Design review of the part shown in the three views and the two pictorial views. Dimensions are in mm from the part's minimum x, y and z. A direction names the side the tool comes from. Give positions to 0.01 mm unless a question says otherwise; leave off trailing zeros. Order: outer loops, then holes, each group sorted by start corner. A loop starts at its lowest first (then second) coordinate and runs counter-clockwise, first axis right, second up. Notation, with made-up numbers: (79.25, 13.5) -> (124.25, 13.5) arc R19 ccw to (124.25, 21.5) -> close; hole circle Ø11 at (70, 71). An arc over 180 degrees is marked (long way). Answer in a Markdown table with one row per item. Add a question column.
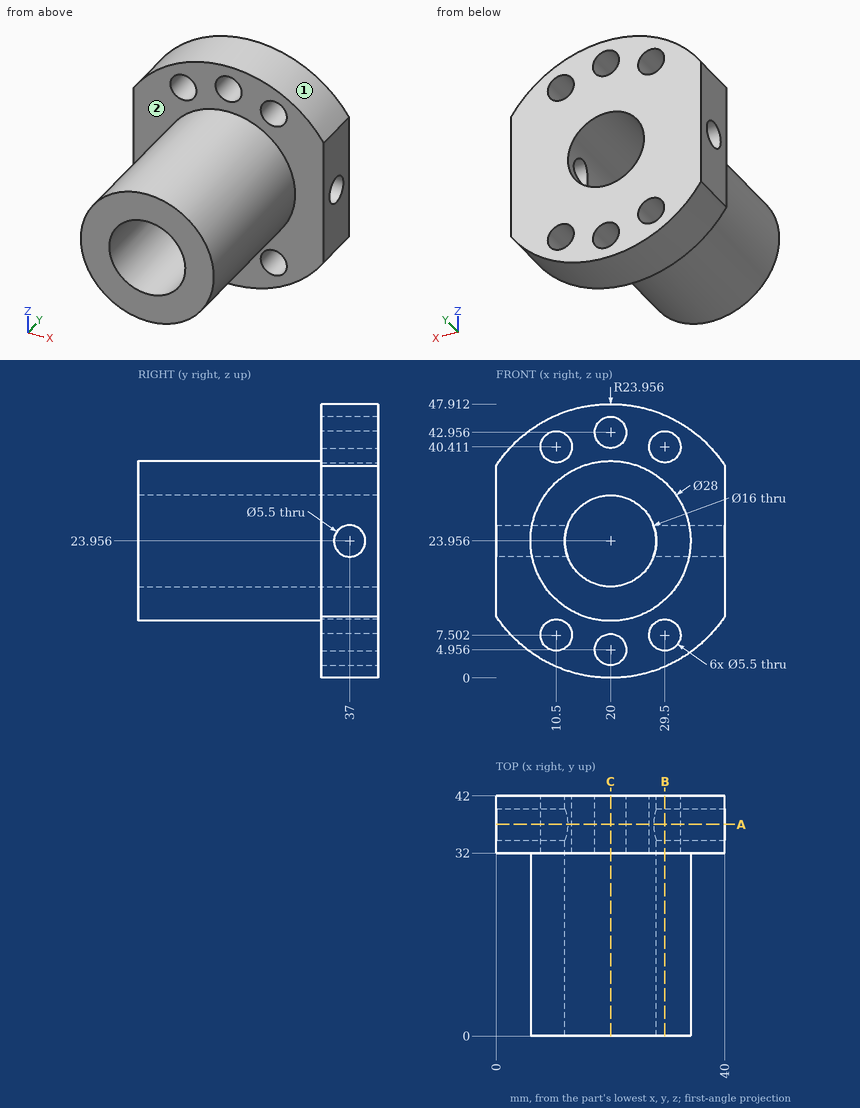
1) Add section A-A, the plane y = 37. Write out the cut boundary in (x, z), and give its area (3 significant figures).
2) For L1, parallel to Z at x = 10, y = 35 (1 decimal); L2, parallel to X at y = 24.5, z = 24.5; L3, parallel to Z at x = 22, y = 12, list the stretches that pass through material, from the lowest coordinate up.
3) Clearance check with flat-ended pins moving along their axes: P1, Ø8, axis at x = 16.5, z = 27, coming from the +Y side; P2, Ø10, axis at y = 10, z = 9.5, coming from the +X side (1 decimal); P3, Ø14.5, axis at x = 20, z = 23.96, coming from the +Y side; P4, Ø6, axis at x = 30, y = 9, coming from the -Z side. State where each tip first meets the part, or that it passes through.
4) Add section C-C, the plane x = 20. Write out the cut boundary in (y, z), and give its area (3 significant figures).
5) Machinability: for the marked faces 1 and 2, which of the approach directions +Z, -Z, +X, -X, +Y, -Y give a long, thin tool a straight path to every point of the face, cutting with its end or side? Answer none if there is none.
6) Add section B-B, the plane x = 29.5. Give the number of separate pieces and of enclosed holes in the cut face, and give its area (3 significant figures).
Verdict:
| question | item | result |
|---|---|---|
| 1 | outline | (0, 10.77) arc R23.96 ccw to (40, 10.77) -> (40, 21.21) -> (27.51, 21.21) arc R8 cw to (12.49, 21.21) -> (0, 21.21) -> close; (0, 26.71) -> (12.49, 26.71) arc R8 cw to (27.51, 26.71) -> (40, 26.71) -> (40, 37.14) arc R23.96 ccw to (0, 37.14) -> close; hole circle Ø5.5 at (10.5, 7.5); hole circle Ø5.5 at (10.5, 40.41); hole circle Ø5.5 at (20, 4.96); hole circle Ø5.5 at (20, 42.96); hole circle Ø5.5 at (29.5, 7.5); hole circle Ø5.5 at (29.5, 40.41) |
| 1 | area | 1,180 mm2 |
| 2 | L1 | z = 2.2 to 4.8, 10.2 to 22.1, 25.8 to 37.7, 43.1 to 45.7 |
| 2 | L2 | x = 6.01 to 12.02, 27.98 to 33.99 |
| 2 | L3 | z = 10.1 to 16.21, 31.7 to 37.81 |
| 3 | P1 | stops at y = 42 |
| 3 | P2 | stops at x = 30.3 |
| 3 | P3 | passes through |
| 3 | P4 | stops at z = 11.83 |
| 4 | outline | (0, 9.96) -> (32, 9.96) -> (32, 7.71) -> (42, 7.71) -> (42, 15.96) -> (0, 15.96) -> close; (0, 31.96) -> (42, 31.96) -> (42, 40.21) -> (32, 40.21) -> (32, 37.96) -> (0, 37.96) -> close; (32, 0) -> (42, 0) -> (42, 2.21) -> (32, 2.21) -> close; (32, 45.71) -> (42, 45.71) -> (42, 47.91) -> (32, 47.91) -> close |
| 4 | area | 593 mm2 |
| 5 | face 1 | +Z, +Y, -Y |
| 5 | face 2 | -Y |
| 6 | separate pieces | 3 |
| 6 | enclosed holes | 1 |
| 6 | area | 964 mm2 |
